from build123d import *

# Parameters (mm, degrees)
F1_DEPTH = 3.175
F2_R     = 63.49999
F3_D     = 5.1054


# Not quite as in the source:
# - a fillet or chamfer is up to 0.001 mm smaller than in the source, because OpenCascade refuses the exact size


with BuildPart() as f1:
    # F0 (on Top) → F1 (new body)
    with BuildSketch(Plane.XY):
        Polygon((-101.6, 0), (0, 0), (0, 101.6), (-38.1, 101.6), (-38.1, 25.4), (-101.6, 25.4), align=None)
    extrude(amount=F1_DEPTH)

    # F2 (radius 63.5 in the source; OpenCascade refuses exactly that, so slightly less here)
    f2_edges = [f1.edges().sort_by_distance(p)[0] for p in [
        (-38.1, 25.4, 1.5875),
    ]]
    fillet(f2_edges, radius=F2_R)

    # F3 (through all)
    with Locations(Plane(origin=(0, 0, 0), x_dir=(1, 0, 0), z_dir=(0, 0, -1))):
        with Locations((-82.55, -12.7), (-57.15, -12.7), (-19.05, -12.7), (-19.05, -44.45)):
            Hole(F3_D / 2)


solid = f1.part
Geometry: final body of the model. Coordinates: model frame, mm. A direction names the side the tool comes from. Give positions to 0.01 mm unless a question says otherwise; leave off trailing zeros. Write each loop counter-clockwise with the first axis right and the second up, starting at its lowest first coordinate (ties: lowest second). Pieces come first, ordered by that corner, then holes. Notation, with made-up numbers: (45, 4) - (65, 4) arc R28 cw to (65, 26) - close; hole circle Ø11 at (-40, -18.75). An arc over 180 degrees is marked (long way). Return JSON: item names as keys, results as strings. Group by question number.
1) Line query: line 1 (Y direction, x = -19.05, z = 2); line 2 (X direction, y = 12.7, z = 1.45); line 3 (Y direction, x = -82.55, z = 0.65). Output: solid intervals per line, ascending.
2) Mould query, pull axis Y, two halves, no side actions, for faces 3 (the flat face through (-19, 101.6, 2)), 4 (the flat face through (-40, 40, 0)), 5 (the cylindrical face through (-54.6, 12.6, 1.6)), 6 (the flat face through (-52, 0, 2)). Classes: released by +Y, released by -Y, zero draft, split by the parting line, or undercut.
3) Section A-A on y = 12.7. Return the cut outline in (x, z) (3 decimals).
4) Section C-C on x = -82.55. Return the cut outline in (y, z) (3 decimals), plus the area to 3 significant figures.
5) First-contact query: P1, Ø4, axis at x = -19.05, y = 44.45, coming from the -Z side; P2, Ø1.6, axis at y = 98, z = 1, coming from the -X side. Flat tips, straight axial feed; report the tip coordinate or a pass-through.
6) Set-up query: faces 1 (the cylindrical face through (-81.997, 15.192, 1.61)), 2 (the flat face through (-38.1, 95, 2)). Return all of +Z, -Z, +X, -X, +Y, -Y with unobstructed straight access to the full face (end or side cutting, diameter ignored); none if empty.
7) Section D-D on x = -57.15. Return the cut outline in (y, z) (3 decimals).
8) Section B-B on z = 0.8. State how many separate pieces and enclosed holes the cut face has, plus the area to 3 significant figures.
Filled in:
{
 "1": {"line 1": "y = 0 to 10.15, 15.25 to 41.9, 47 to 101.6", "line 2": "x = -101.6 to -85.1, -80 to -59.7, -54.6 to -21.6, -16.5 to 0", "line 3": "y = 0 to 10.15, 15.25 to 28.32"},
 "2": {"face 3": "released by +Y", "face 4": "zero draft", "face 5": "undercut", "face 6": "released by -Y"},
 "3": {"outline": "(-101.6, 0) - (-85.103, 0) - (-85.103, 3.175) - (-101.6, 3.175) - close; (-79.997, 0) - (-59.703, 0) - (-59.703, 3.175) - (-79.997, 3.175) - close; (-54.597, 0) - (-21.603, 0) - (-21.603, 3.175) - (-54.597, 3.175) - close; (-16.497, 0) - (0, 0) - (0, 3.175) - (-16.497, 3.175) - close"},
 "4": {"outline": "(0, 0) - (10.147, 0) - (10.147, 3.175) - (0, 3.175) - close; (15.253, 0) - (28.325, 0) - (28.325, 3.175) - (15.253, 3.175) - close", "area": "73.7 mm^2"},
 "5": {"P1": "passes through", "P2": "stops at x = -38.1"},
 "6": {"face 1": "+Z, -Z", "face 2": "+Z, -Z, -X, +Y"},
 "7": {"outline": "(0, 0) - (10.147, 0) - (10.147, 3.175) - (0, 3.175) - close; (15.253, 0) - (43.552, 0) - (43.552, 3.175) - (15.253, 3.175) - close"},
 "8": {"separate pieces": "1", "enclosed holes": "4", "area": "6,270 mm^2"}
}
